from build123d import *

# Parameters (mm, degrees)
F0_W     = 20
F0_H     = 7
F1_DEPTH = 40
F2_W     = 7
F2_H     = 10
F3_DEPTH = 10


with BuildPart() as f1:
    # F0 (on Top) → F1 (new body)
    with BuildSketch(Plane.XY):
        with Locations((-20, -13.28286)):
            Rectangle(F0_W, F0_H)
    extrude(amount=F1_DEPTH)

    # F2 (on face) → F3 (join)
    with BuildSketch(Plane.YZ.offset(-10)):
        with Locations((-13.28286, 35)):
            Rectangle(F2_W, F2_H)
        with Locations((-13.28286, 15)):
            Rectangle(F2_W, F2_H)
    extrude(amount=F3_DEPTH)


solid = f1.part
Design review of the part built by this model. Coordinates are the model's own, in mm. A direction names the side the tool comes from. Coordinates: 2 decimals unless noted, no trailing zeros. Write each loop counter-clockwise with the first axis right and the second up, starting at its lowest first coordinate (ties: lowest second). Pieces come first, ordered by that corner, then holes. Notation, with made-up numbers: (-30, -38) -> (17, -38) arc R20 ccw to (17, 1) -> close; hole circle Ø7 at (56.25, 42). An arc over 180 degrees is marked (long way). Write each question's results on one line, items separated by ' | '. Start each with the question number.
(1) Take a section at A-A on x = -3. Write out the cut boundary in (y, z), and give its area (3 significant figures).
(2) Take a section at C-C on z = 27.5. Write out the cut boundary in (x, y), and give its area (3 significant figures).
(3) Tool access review of faces 4 (the face through (-10, -13, 25)), 5 (the face through (0, -13, 35)), 6 (the face through (-10, -13, 5)): name each direction out of +Z, -Z, +X, -X, +Y, -Y from which nothing blocks a thin tool from reaching the whole face with its end or side.
(4) Take a section at B-B on y = -12.5. Write out the cut boundary in (x, z), and give its area (3 significant figures).
(5) The part is to be moulded in two halves that separate along Z. For faces 1 (the face through (-20, -13, 0)), 2 (the face through (0, -13, 15)), 3 (the face through (-5, -13, 20)), say which applies: pulls with the +Z half, pulls with the -Z half, needs draft (parallel to the pull), parting line crosses it, or undercut.
(6) For line 1 along Z through (x, y) = (-6, -13); line 2 along X through (y, z) = (-12.5, 24.5), list the stretches that pass through material, from the lowest coordinate up. Write a range as from..to.
(7) Clearance check with a flat-ended pin moving along its axis: P1, Ø3.5, axis at x = -5.5, y = -12, coming from the -Z side. State where the tip first meets the part, or that it passes through.
Results found:
1) outline: (-16.78, 10) -> (-9.78, 10) -> (-9.78, 20) -> (-16.78, 20) -> close; (-16.78, 30) -> (-9.78, 30) -> (-9.78, 40) -> (-16.78, 40) -> close | area: 140 mm2
2) outline: (-30, -16.78) -> (-10, -16.78) -> (-10, -9.78) -> (-30, -9.78) -> close | area: 140 mm2
3) face 4: +X, +Y, -Y | face 5: +Z, -Z, +X, +Y, -Y | face 6: -Z, +X, +Y, -Y
4) outline: (-30, 0) -> (-10, 0) -> (-10, 10) -> (0, 10) -> (0, 20) -> (-10, 20) -> (-10, 30) -> (0, 30) -> (0, 40) -> (-30, 40) -> close | area: 1,000 mm2
5) face 1: pulls with the -Z half | face 2: needs draft | face 3: undercut
6) line 1: z = 10..20, 30..40 | line 2: x = -30..-10
7) P1: stops at z = 10
